Source: CAD feature listing. Evaluate the final solid. Frame: model axes, mm. A direction names the side the tool comes from. Give positions to 0.01 mm unless a question says otherwise; leave off trailing zeros. Write each loop counter-clockwise with the first axis right and the second up, starting at its lowest first coordinate (ties: lowest second). Pieces come first, ordered by that corner, then holes. Notation, with made-up numbers: (-24.75, 88) - (3.25, 88) arc R22 ccw to (3.25, 109) - close; hole circle Ø5 at (2, -31.75). An arc over 180 degrees is marked (long way). Answer as a JSON object with one key per item and string values. Group by question number.
from build123d import *

# Parameters (mm, degrees)
SKETCH1_W               = 41
SKETCH1_H               = 34.5
SKETCH1_W_2             = 35
SKETCH1_H_2             = 28.5
BOSS_EXTRUDE1_DEPTH     = 5
SKETCH2_W               = 35
SKETCH2_H               = 28.5
BOSS_EXTRUDE2_DEPTH     = 1
SKETCH6_W               = 34.5
SKETCH6_H               = 5
CUT_EXTRUDE2_DEPTH      = 3
SKETCH7_W               = 1.6
SKETCH7_H               = 3
BOSS_EXTRUDE3_DEPTH     = 4
CHAMFER1_SIZE           = 3
SKETCH14_W              = 3.502632447
SKETCH14_H              = 20.452559449
CUT_EXTRUDE6_DEPTH      = 10
BOSS_EXTRUDE5_DEPTH     = 4
BOSS_EXTRUDE7_DEPTH     = 1
SKETCH9_W               = 3.28281374
SKETCH9_H               = 22.420706044
CUT_EXTRUDE3_DEPTH      = 4
BOSS_EXTRUDE4_DEPTH     = 2
SKETCH12_W              = 3.28281374
SKETCH12_H              = 22.420706044
CUT_EXTRUDE4_DEPTH      = 1
BOSS_EXTRUDE8_DEPTH     = 2
BOSS_EXTRUDE9_DEPTH     = 2
CUT_EXTRUDE7_DEPTH      = 1
CUT_EXTRUDE7_DEPTH_BACK = 4
CHAMFER2_SIZE           = 3
CHAMFER2_EDGE_2_SIZE2   = 3
CHAMFER2_EDGE_2_SIZE    = 3.001586398
CHAMFER3_SIZE           = 2
CUT_EXTRUDE8_DEPTH      = 10
SKETCH29_W              = 2.811538377
SKETCH29_H              = 2
CUT_EXTRUDE9_DEPTH      = 10
SKETCH31_W              = 5.26
SKETCH31_H              = 2
CUT_EXTRUDE10_DEPTH     = 10
SKETCH33_W              = 1.99335007
SKETCH33_H              = 8.633384354
CUT_EXTRUDE11_DEPTH     = 10
FILLET1_R               = 2


with BuildPart() as part:
    # Sketch1 → Boss-Extrude1 (new body)
    with BuildSketch(Plane(origin=(0, 0, 0), x_dir=(1, 0, 0), z_dir=(0, 1, 0))):
        with Locations((-14.14154724, 0.334775681)):
            Rectangle(SKETCH1_W, SKETCH1_H)
        with Locations((-14.14154724, 0.334775681)):
            Rectangle(SKETCH1_W_2, SKETCH1_H_2, mode=Mode.SUBTRACT)
    extrude(amount=BOSS_EXTRUDE1_DEPTH)

    # Sketch2 → Boss-Extrude2 (add)
    with BuildSketch(Plane(origin=(0, 0, 0), x_dir=(1, 0, 0), z_dir=(0, 1, 0))):
        with Locations((-14.14154724, 0.334775681)):
            Rectangle(SKETCH2_W, SKETCH2_H)
    extrude(amount=BOSS_EXTRUDE2_DEPTH)

    # Sketch6 → Cut-Extrude2 (cut)
    with BuildSketch(Plane.ZY.offset(34.64154724)):
        with Locations((-0.334775681, 2.5)):
            Rectangle(SKETCH6_W, SKETCH6_H)
    extrude(amount=-CUT_EXTRUDE2_DEPTH, mode=Mode.SUBTRACT)

    # Sketch7 → Boss-Extrude3 (add)
    with BuildSketch(Plane(origin=(0, 1, 0), x_dir=(1, 0, 0), z_dir=(0, 1, 0))):
        with Locations((-30.84154724, 13.084775681)):
            Rectangle(SKETCH7_W, SKETCH7_H)
        with Locations((-30.84154724, -12.415224319)):
            Rectangle(SKETCH7_W, SKETCH7_H)
    extrude(amount=BOSS_EXTRUDE3_DEPTH)

    # Chamfer1
    chamfer1_edges = [part.edges().sort_by_distance(p)[0] for p in [
        (-31.64154724, 2.5, -17.584775681),
        (-31.64154724, 2.5, 16.915224319),
        (6.35845276, 2.5, -17.584775681),
        (6.35845276, 2.5, 16.915224319),
    ]]
    chamfer(chamfer1_edges, length=CHAMFER1_SIZE)

    # Sketch14 → Cut-Extrude6 (cut)
    with BuildSketch(Plane(origin=(0, 1, 0), x_dir=(1, 0, 0), z_dir=(0, 1, 0))):
        with Locations((5.109768984, -7.134544415)):
            Rectangle(SKETCH14_W, SKETCH14_H)
    extrude(amount=CUT_EXTRUDE6_DEPTH, mode=Mode.SUBTRACT)

    # Sketch17 → Boss-Extrude5 (add)
    with BuildSketch(Plane(origin=(0, 1, 0), x_dir=(1, 0, 0), z_dir=(0, 1, 0))):
        Polygon((3.35845276, 3.09173531), (7.910000942, 0), (7.910000942, -13.915224319), (3.35845276, -13.915224319), (3.35845276, -16.915224319), (10.910000942, -16.915224319), (10.910000942, 3.419581668), (3.35845276, 8.549130391), align=None)
    extrude(amount=BOSS_EXTRUDE5_DEPTH)

    # Sketch19 → Boss-Extrude7 (add)
    with BuildSketch(Plane.XZ):
        Polygon((3.35845276, 16.915224319), (10.910000942, 16.915224319), (10.910000942, -3.419581668), (6.35845276, -6.511316978), (6.35845276, 13.915224319), align=None)
    extrude(amount=-BOSS_EXTRUDE7_DEPTH)

    # Sketch9 → Cut-Extrude3 (cut)
    with BuildSketch(Plane(origin=(0, 1, 0), x_dir=(1, 0, 0), z_dir=(0, 1, 0))):
        with Locations((-30.00014037, 0.374422659)):
            Rectangle(SKETCH9_W, SKETCH9_H)
    extrude(amount=-CUT_EXTRUDE3_DEPTH, mode=Mode.SUBTRACT)

    # Sketch11 → Boss-Extrude4 (add)
    with BuildSketch(Plane.XZ):
        Polygon((-26.665503706, 18.915224319), (-31.64154724, 13.915224319), (-31.64154724, -14.584775681), (-26.629189212, -19.584775681), (4.233785533, -19.584775681), (8.35845276, -15.460108453), (8.35845276, 14.743651444), (4.263960312, 18.915224319), align=None)
    extrude(amount=BOSS_EXTRUDE4_DEPTH)

    # Sketch12 → Cut-Extrude4 (cut)
    with BuildSketch(Plane(origin=(0, 0, 0), x_dir=(1, 0, 0), z_dir=(0, 1, 0))):
        with Locations((-30.00014037, 0.374422659)):
            Rectangle(SKETCH12_W, SKETCH12_H)
    extrude(amount=-CUT_EXTRUDE4_DEPTH, mode=Mode.SUBTRACT)

    # Sketch20 → Boss-Extrude8 (add)
    with BuildSketch(Plane.XZ):
        Polygon((6.227005221, 16.915224319), (10.910000942, 16.915224319), (10.910000942, -3.419581668), (8.35845276, -5.152774704), (8.35845276, 14.743651444), align=None)
    extrude(amount=BOSS_EXTRUDE8_DEPTH)

    # Sketch21 → Boss-Extrude9 (add)
    with BuildSketch(Plane(origin=(0, 0, 0), x_dir=(1, 0, 0), z_dir=(0, 1, 0))):
        Polygon((8.35845276, 7.570549944), (8.35845276, 5.152774704), (10.90766939, 3.421165424), (10.90766939, -16.912751148), (6.227005221, -16.915224319), (4.263960312, -18.915224319), (7.06681334, -18.91478086), (12.90766939, -18.911694666), (12.90766939, 4.480398389), align=None)
    extrude(amount=-BOSS_EXTRUDE9_DEPTH)

    # Sketch23 → Cut-Extrude7 (cut, two sides)
    with BuildSketch(Plane(origin=(0, 5, 0), x_dir=(1, 0, 0), z_dir=(0, 1, 0))) as cut_extrude7_sk:
        Polygon((7.910000942, 0), (7.910000942, 1.828776855), (3.35845276, 4.913740582), (3.35845276, 3.09173531), align=None)
    extrude(amount=CUT_EXTRUDE7_DEPTH, mode=Mode.SUBTRACT)
    extrude(cut_extrude7_sk.sketch, amount=-CUT_EXTRUDE7_DEPTH_BACK, mode=Mode.SUBTRACT)

    # Chamfer2
    chamfer2_edges = [part.edges().sort_by_distance(p)[0] for p in [
        (10.910000942, 2.5, 16.915224319),
    ]]
    chamfer(chamfer2_edges, length=CHAMFER2_SIZE)

    # Chamfer2 edge 2
    chamfer2_edge_2_edges = [part.edges().sort_by_distance(p)[0] for p in [
        (12.90766939, -1, 18.911694666),
    ]]
    chamfer(chamfer2_edge_2_edges, length=CHAMFER2_EDGE_2_SIZE, length2=CHAMFER2_EDGE_2_SIZE2)

    # Chamfer3
    chamfer3_edges = [part.edges().sort_by_distance(p)[0] for p in [
        (7.910000942, 3, 13.915224319),
    ]]
    chamfer(chamfer3_edges, length=CHAMFER3_SIZE)

    # Sketch27 → Cut-Extrude8 (cut)
    with BuildSketch(Plane(origin=(0, 0, 0), x_dir=(1, 0, 0), z_dir=(0, 1, 0))):
        Polygon((-23.564566169, -18.915224319), (-23.564566169, -16.956730787), (-23.564566169, -16.915224319), (-28.64154724, -16.915224319), (-26.665503706, -18.915224319), align=None)
    extrude(amount=-CUT_EXTRUDE8_DEPTH, mode=Mode.SUBTRACT)

    # Sketch29 → Cut-Extrude9 (cut)
    with BuildSketch(Plane(origin=(-22.95033658, 0, 22.675432092), x_dir=(-0.702833562, 0, -0.711354331), z_dir=(0.711354331, 0, -0.702833562))):
        with Locations((6.691753419, -1)):
            Rectangle(SKETCH29_W, SKETCH29_H)
    extrude(amount=-CUT_EXTRUDE9_DEPTH, mode=Mode.SUBTRACT)

    # Sketch31 → Cut-Extrude10 (cut)
    with BuildSketch(Plane(origin=(0, 0, 0), x_dir=(1, 0, 0), z_dir=(0, 1, 0))):
        with Locations((-26.164712617, 18.586994213)):
            Rectangle(SKETCH31_W, SKETCH31_H)
    extrude(amount=-CUT_EXTRUDE10_DEPTH, mode=Mode.SUBTRACT)

    # Sketch33 → Cut-Extrude11 (cut)
    with BuildSketch(Plane.XZ.offset(2)):
        with Locations((11.910994355, 5.861564698)):
            Rectangle(SKETCH33_W, SKETCH33_H)
    extrude(amount=-CUT_EXTRUDE11_DEPTH, mode=Mode.SUBTRACT)

    # Fillet1
    fillet1_edges = [part.edges().sort_by_distance(p)[0] for p in [
        (4.233785533, -1, -19.584775681),
        (8.35845276, -1, -15.460108453),
        (8.35845276, -1, -7.570549944),
        (12.90766939, -1, -4.480398389),
        (9.906083411, -1, 18.913280645),
        (12.90766939, -1, 15.911694666),
    ]]
    fillet(fillet1_edges, radius=FILLET1_R)


solid = part.part
Q1. Draft query along Z for faces 1 (the flat face through (-31.642, -1.3, -0.3)), 2 (the flat face through (-10, -1, -19.585)), 3 (the flat face through (3.358, 3, -10)). Return one class per face: released by +Z, released by -Z, zero draft, split by the parting line, or undercut.
Q2. First-contact query: pin 1 Ø0.8 at (x, y) = (-31, 3.5) entering from -Z; pin 2 Ø3 at (x, y) = (-19, 3.5) entering from +Z; pin 3 Ø1.6 at (y, z) = (-1, -12.5) entering from +X. Flat tips, straight axial feed; report the tip coordinate or a pass-through.
Q3. Section B-B on y = 3.25. Return the cut outline in (x, z).
Q4. Section A-A on z = 0. Return the cut outline in (x, y).
Q5. Section C-C on x = -15. Return the cut outline in (y, z), then the cut area to 4 significant figures.
Q6. Ray query, probe 1 along Z at (x, y) = (-5, 2); probe 2 along X at (y, z) = (1.5, 11); probe 3 along X at (y, z) = (2.25, -12). Return the intervals inside material, ascending. Write a range as [from, to].
Q7. Reachability of faces 4 (the flat face through (-12, 3, 13.915)), 5 (the flat face through (-13, 2, -17.585)), 6 (the flat face through (4.837, 2.465, -16.106)), 7 (the flat face through (8.358, -1, -12)), 8 (the flat face through (5.666, 3.028, -3.35)) from +Z, -Z, +X, -X, +Y, -Y: full face, straight path, thin tool, end or side. Return the list, or none.
Taken from the geometry:
{
 "1": {"face 1": "zero draft", "face 2": "released by -Z", "face 3": "undercut"},
 "2": {"pin 1": "stops at z = -15.63", "pin 2": "stops at z = 16.92", "pin 3": "stops at x = 8.36"},
 "3": {"outline": "(-31.64, -14.58) - (-28.64, -17.58) - (3.36, -17.58) - (6.36, -14.58) - (6.36, -6.51) - (10.91, -3.42) - (10.91, 13.92) - (7.91, 16.92) - (-28.64, 16.92) - (-31.64, 13.92) - (-31.64, 10.92) - (-30.04, 10.92) - (-30.04, 13.92) - (5.91, 13.92) - (7.91, 11.92) - (7.91, -1.83) - (3.36, -4.91) - (3.36, -14.58) - (-30.04, -14.58) - (-30.04, -11.58) - (-31.64, -11.58) - close"},
 "4": {"outline": "(-31.64, -2) - (12.91, -2) - (12.91, 0) - (10.91, 0) - (10.91, 5) - (7.91, 5) - (7.91, 1) - (-28.36, 1) - (-28.36, -1) - (-31.64, -1) - close"},
 "5": {"outline": "(-2, -19.58) - (0, -19.58) - (0, -17.58) - (5, -17.58) - (5, -14.58) - (1, -14.58) - (1, 13.92) - (5, 13.92) - (5, 16.92) - (0, 16.92) - (0, 18.92) - (-2, 18.92) - close", "area": "135.5 mm²"},
 "6": {"probe 1": "z = [-17.58, -14.58], [13.92, 16.92]", "probe 2": "x = [-31.64, -30.04], [7.91, 10.91]", "probe 3": "x = [-31.64, -30.04], [3.36, 6.36]"},
 "7": {"face 4": "+Y", "face 5": "-Z, +X, -X, +Y", "face 6": "-Z, +X, +Y", "face 7": "-Z, +X, +Y, -Y", "face 8": "-X, +Y"}
}
